CAD build for the part. Positions are in the model's coordinates, mm. Round coordinates to 2 decimals unless told otherwise and drop trailing zeros. Write each loop counter-clockwise with the first axis right and the second up, starting at its lowest first coordinate (ties: lowest second). Pieces come first, ordered by that corner, then holes. Notation, with made-up numbers: (35.25, 40.5) -> (92.25, 40.5) arc R30 ccw to (92.25, 65.5) -> close; hole circle Ø6 at (21.25, 17.25). An arc over 180 degrees is marked (long way). Put each result on its own line as item: value. Start each with the question number.
1. Pull direction Y, two halves, no side cores. Call faces 1 (the cylindrical face through (2.1, 16.52, -1.51)), 2 (the cylindrical face through (-0.395, 12.676, -1.485)), 3 (the flat face through (-2.8, 0, -1)): pulls with the +Y half, pulls with the -Y half, needs draft (parallel to the pull), parting line crosses it, or undercut.
2. Saw through at A-A on x = 0. List the corners of the cut face in (y, z), and give its area (3 significant figures).
3. Flat gauge pin, fed straight in: P1, Ø2, axis at x = 0, y = 14.45, coming from the -Z side. Where does the tip first touch, or does it go through?
4. Drill centre lines: line 1 (Y direction, x = 0, z = -1.3); line 2 (X direction, y = -15, z = -0.9); line 3 (Y direction, x = -0.7, z = -0.65). Where is each one in solid material? Low to high. Write a range as from..to.
5. Saw through at B-B on z = -1.55. List the corners of the cut face in (x, y).
from build123d import *

# Parameters (mm, degrees)
SKETCH1_W           = 50
SKETCH1_H           = 8
SKETCH1_R           = 1.5
SKETCH1_R_2         = 2.6
BOSS_EXTRUDE1_DEPTH = 3
FILLET1_R           = 3.5
SCALE1_SCALE        = 0.7


with BuildPart() as part:
    # Sketch1 → Boss-Extrude1 (new body)
    with BuildSketch(Plane(origin=(0, 0, 0), x_dir=(0, 1, 0), z_dir=(0, 0, 1))):
        Rectangle(SKETCH1_W, SKETCH1_H)
        with Locations(Location((-21, 0, 0), (0, 0, 270))):
            Circle(SKETCH1_R, mode=Mode.SUBTRACT)
        with Locations(Location((21, 0, 0), (0, 0, 270))):
            Circle(SKETCH1_R_2, mode=Mode.SUBTRACT)
    extrude(amount=-BOSS_EXTRUDE1_DEPTH)

    # Fillet1
    fillet1_edges = [part.edges().sort_by_distance(p)[0] for p in [
        (4, 25, -1.5),
        (4, -25, -1.5),
        (-4, -25, -1.5),
        (-4, 25, -1.5),
    ]]
    fillet(fillet1_edges, radius=FILLET1_R)


with BuildPart() as part_1:
    # Scale1: scaled about (0, -0.82380326, -1.5)
    add(part.part.scale(SCALE1_SCALE).moved(Location((0, -0.247140978, -0.45))))


solid = part_1.part
Return value:
1. face 1: pulls with the +Y half
1. face 2: undercut
1. face 3: needs draft
2. outline: (-17.75, -2.55) -> (-16, -2.55) -> (-16, -0.45) -> (-17.75, -0.45) -> close; (-13.9, -2.55) -> (12.63, -2.55) -> (12.63, -0.45) -> (-13.9, -0.45) -> close; (16.27, -2.55) -> (17.25, -2.55) -> (17.25, -0.45) -> (16.27, -0.45) -> close
2. area: 61.4 mm^2
3. P1: passes through
4. line 1: y = -17.75..-16, -13.9..12.63, 16.27..17.25
4. line 2: x = -2.8..-1.05, 1.05..2.8
4. line 3: y = -17.72..-15.73, -14.16..12.77, 16.13..17.23
5. outline: (-2.8, -15.3) arc R2.45 ccw to (-0.35, -17.75) -> (0.35, -17.75) arc R2.45 ccw to (2.8, -15.3) -> (2.8, 14.8) arc R2.45 ccw to (0.35, 17.25) -> (-0.35, 17.25) arc R2.45 ccw to (-2.8, 14.8) -> close; hole circle Ø3.64 at (0, 14.45); hole circle Ø2.1 at (0, -14.95)
